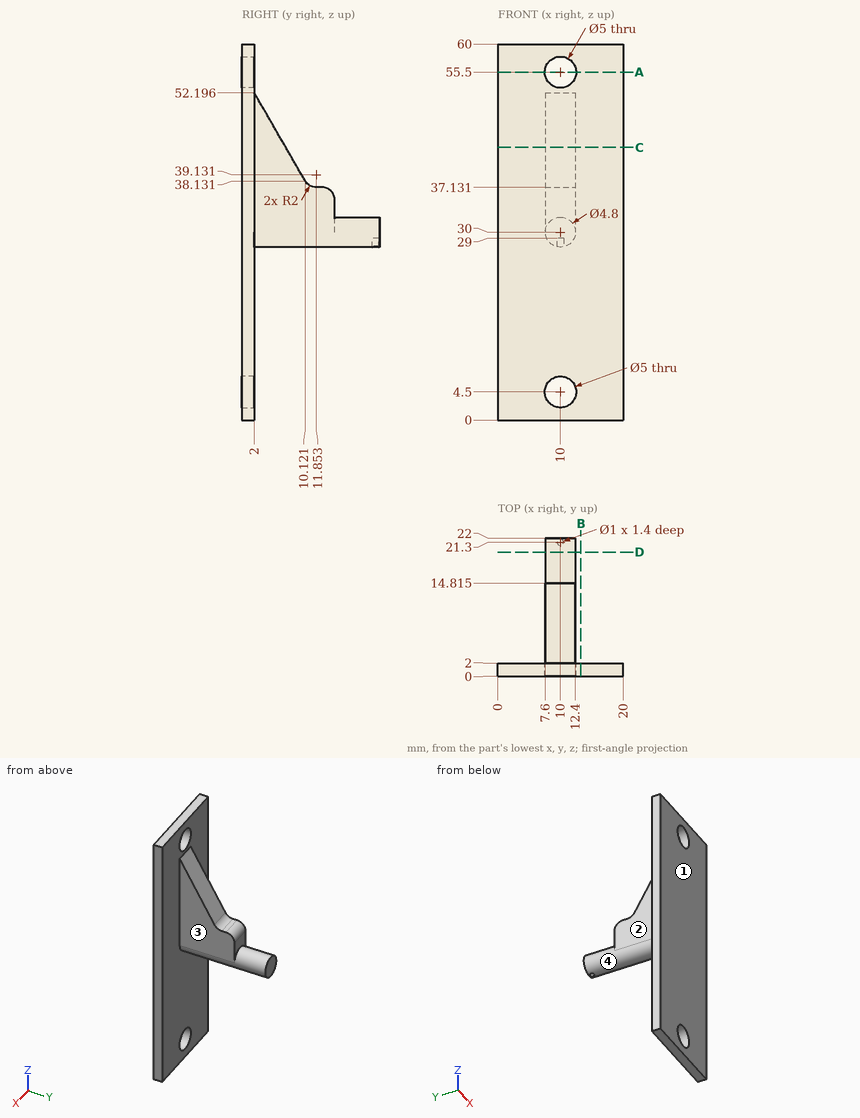
Verification items for this drawing (mm, ordinates from the low corner). A direction names the side the tool comes from. Give positions to 0.01 mm unless a question says otherwise; leave off trailing zeros. Write each loop counter-clockwise with the first axis right and the second up, starting at its lowest first coordinate (ties: lowest second). Pieces come first, ordered by that corner, then holes.
1) Cross-section at A-A (z = 55.5). Record the boundary of the cut face in (x, y), plus the area to 3 significant figures.
Values follow:
outline: (0, 0) - (7.5, 0) - (7.5, 2) - (0, 2) - close; (12.5, 0) - (20, 0) - (20, 2) - (12.5, 2) - close
area: 30.0 mm2
2) Cross-section at B-B (x = 13.25). Record the boundary of the cut face in (y, z).
Values follow:
outline: (0, 0) - (2, 0) - (2, 60) - (0, 60) - close
3) Thickness scan on line 1 (X direction, y = 0.5, z = 4.5); line 2 (X direction, y = 21.3, z = 28.1) (1 decimal); line 3 (Y direction, x = 13.25, z = 16). Record the ranges inside material, lowest first.
Values follow:
line 1: x = 0 to 7.5, 12.5 to 20
line 2: x = 8.5 to 9.5, 10.5 to 11.5
line 3: y = 0 to 2
4) Cross-section at C-C (z = 43.5). Record the boundary of the cut face in (x, y).
Values follow:
outline: (0, 0) - (20, 0) - (20, 2) - (12.4, 2) - (12.4, 7.02) - (7.6, 7.02) - (7.6, 2) - (0, 2) - close
5) Set-up check for the marked faces 1, 2, 3 and 4: record each of +Z, -Z, +X, -X, +Y, -Y from which the full face is reachable in a straight line by a thin tool's end or side.
Values follow:
face 1: +Z, -Z, +X, -X, -Y
face 2: +Z, -Z, -X, +Y
face 3: +Z, -Z, +X, +Y
face 4: +Y
6) Go/stop test with flat-tipped pins: pin 1 Ø3 at (y, z) = (5.5, 53) entering from -X; pin 2 Ø12 at (x, z) = (6, 22.5) entering from +Y; pin 3 Ø10.5 at (y, z) = (11.5, 39.5) entering from +X; pin 4 Ø0.8 at (x, y) = (10, 21) entering from -Z. Record where each tip stops, or that it passes through.
Values follow:
pin 1: passes through
pin 2: stops at y = 2
pin 3: stops at x = 12.4
pin 4: stops at z = 27.6
7) Cross-section at D-D (y = 19.75). Record the boundary of the cut face in (x, z), plus the area to 3 significant figures.
Values follow:
outline: circle Ø4.8 at (10, 30)
area: 18.1 mm2
